Model file for the job. Use its own axes, mm. Face numbers are marked on the shaded views. Give positions to 0.01 mm unless a question says otherwise; leave off trailing zeros. Order: outer loops, then holes, each group sorted by start corner. A loop starts at its lowest first (then second) coordinate and runs counter-clockwise, first axis right, second up. Notation, with made-up numbers: M 79,33 L 125,33 A22 ccw 125,65 Z; hole C 72,-15.75 d7. An arc over 180 degrees is marked long. Return JSON: item names as keys, results as strings. Group by question number.
1. Slice it at A-A on y = -5. List the corners of the cut face in (x, z) (3 decimals).
2. Pin check, flat tips, straight feed: pin 1 (2 mm diameter, centred on x = 0.5, y = -42.5, fed in from +Z) (3 decimals); pin 2 (1.5 mm diameter, centred on y = -15.5, z = 0, fed in from +X) (3 decimals); pin 3 (1.5 mm diameter, centred on x = -2, y = -32.5, fed in from +Z). Stop position of each tip, or through.
3. Wall check: probe 1 along X at (y, z) = (-32.5, 0) (3 decimals); probe 2 along Y at (x, z) = (2.25, 1); probe 3 along Y at (x, z) = (0, 2.5). Give the ranges that are in metal, low to high. Write a range as [from, to].
4. Two-plate mould, pull along X, no slides. Class the marked faces 1 and 2: released by +X, released by -X, zero draft, split by the parting line, or undercut.
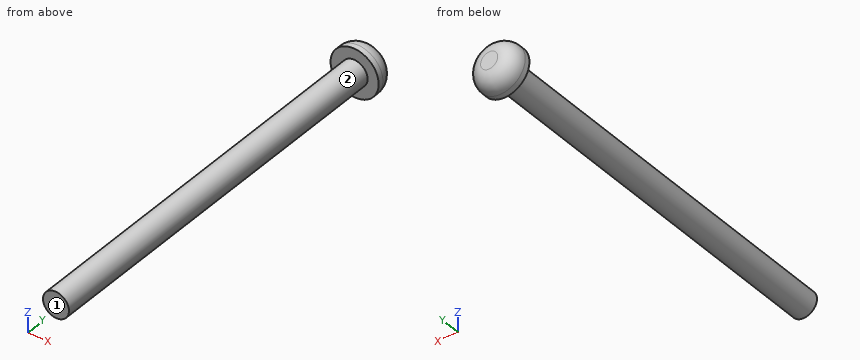
from build123d import *

# Parameters (mm, degrees)
CROQUIS1_R              = 1.675
SALIENTE_EXTRUIR1_DEPTH = 49.65
CROQUIS2_R              = 3.1
SALIENTE_EXTRUIR2_DEPTH = 2.7
REDONDEO1_R             = 2


with BuildPart() as part:
    # Croquis1 → Saliente-Extruir1 (new body)
    with BuildSketch(Plane(origin=(0, 0, 0), x_dir=(1, 0, 0), z_dir=(0, 1, 0))):
        with Locations(Location((0, 0, 0), (0, 0, 270))):
            Circle(CROQUIS1_R)
    extrude(amount=-SALIENTE_EXTRUIR1_DEPTH)

    # Croquis2 → Saliente-Extruir2 (add)
    with BuildSketch(Plane(origin=(0, 0, 0), x_dir=(1, 0, 0), z_dir=(0, 1, 0))):
        with Locations(Location((0, 0, 0), (0, 0, 90))):
            Circle(CROQUIS2_R)
    extrude(amount=SALIENTE_EXTRUIR2_DEPTH)

    # Redondeo1
    redondeo1_edges = [part.edges().sort_by_distance(p)[0] for p in [
        (0, 2.7, 3.1),
    ]]
    fillet(redondeo1_edges, radius=REDONDEO1_R)


solid = part.part
Result:
{
 "1": {"outline": "C 0,0 d3.35"},
 "2": {"pin 1": "stops at z = 1.675", "pin 2": "stops at x = 1.675", "pin 3": "stops at z = 1.11"},
 "3": {"probe 1": "x = [-1.675, 1.675]", "probe 2": "y = [0, 2.16]", "probe 3": "y = [0, 2.13]"},
 "4": {"face 1": "zero draft", "face 2": "split by the parting line"}
}
